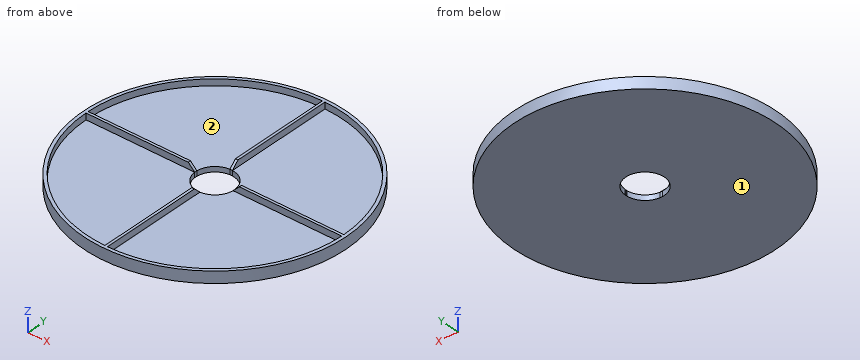
```python
from build123d import *

# Parameters (mm, degrees)
F1_DEPTH = 4
F0_R     = 102.5
F2_DEPTH = 9
F3_SIZE  = 5


with BuildPart() as f1:
    # F0 (on Top) → F1 (new body)
    with BuildSketch(Plane.XY):
        with BuildLine():
            Line((-1, -99.994999875), (-1, -14.9666295471))
            ThreePointArc((-1, -14.9666295471), (-10.6066017178, -10.6066017178), (-14.9666295471, -1))
            Line((-14.9666295471, -1), (-99.994999875, -1))
            ThreePointArc((-99.994999875, -1), (-70.7106781187, -70.7106781187), (-1, -99.994999875))
        make_face()
    extrude(amount=F1_DEPTH)



with BuildPart() as f1b:
    # F0 (on Top) → F1, piece 2 (new body)
    with BuildSketch(Plane.XY):
        with BuildLine():
            Line((99.994999875, -1), (14.9666295471, -1))
            ThreePointArc((14.9666295471, -1), (10.6066017178, -10.6066017178), (1, -14.9666295471))
            Line((1, -14.9666295471), (1, -99.994999875))
            ThreePointArc((1, -99.994999875), (70.7106781187, -70.7106781187), (99.994999875, -1))
        make_face()
    extrude(amount=F1_DEPTH)


with BuildPart() as f1c:
    # F0 (on Top) → F1, piece 3 (new body)
    with BuildSketch(Plane.XY):
        with BuildLine():
            ThreePointArc((1, 14.9666295471), (10.6066017178, 10.6066017178), (14.9666295471, 1))
            Line((14.9666295471, 1), (99.994999875, 1))
            ThreePointArc((99.994999875, 1), (70.7106781187, 70.7106781187), (1, 99.994999875))
            Line((1, 99.994999875), (1, 14.9666295471))
        make_face()
    extrude(amount=F1_DEPTH)


with BuildPart() as f1d:
    # F0 (on Top) → F1, piece 4 (new body)
    with BuildSketch(Plane.XY):
        with BuildLine():
            ThreePointArc((-14.9666295471, 1), (-10.6066017178, 10.6066017178), (-1, 14.9666295471))
            Line((-1, 14.9666295471), (-1, 99.994999875))
            ThreePointArc((-1, 99.994999875), (-70.7106781187, 70.7106781187), (-99.994999875, 1))
            Line((-99.994999875, 1), (-14.9666295471, 1))
        make_face()
    extrude(amount=F1_DEPTH)


with BuildPart() as f1_1:
    add(f1.part)

    add(f1b.part)  # F2 merges F1b

    add(f1c.part)  # F2 merges F1c

    add(f1d.part)  # F2 merges F1d
    # F0 (on Top) → F2 (join)
    with BuildSketch(Plane.XY):
        Circle(F0_R)
        with BuildLine():
            ThreePointArc((14.9666295471, 1), (14.9916550655, 0.5002783193), (15, 0))
            ThreePointArc((15, 0), (14.9916550655, -0.5002783193), (14.9666295471, -1))
            Line((14.9666295471, -1), (99.994999875, -1))
            ThreePointArc((99.994999875, -1), (70.7106781187, -70.7106781187), (1, -99.994999875))
            Line((1, -99.994999875), (1, -14.9666295471))
            ThreePointArc((1, -14.9666295471), (0, -15), (-1, -14.9666295471))
            Line((-1, -14.9666295471), (-1, -99.994999875))
            ThreePointArc((-1, -99.994999875), (-70.7106781187, -70.7106781187), (-99.994999875, -1))
            Line((-99.994999875, -1), (-14.9666295471, -1))
            ThreePointArc((-14.9666295471, -1), (-15, 0), (-14.9666295471, 1))
            Line((-14.9666295471, 1), (-99.994999875, 1))
            ThreePointArc((-99.994999875, 1), (-70.7106781187, 70.7106781187), (-1, 99.994999875))
            Line((-1, 99.994999875), (-1, 14.9666295471))
            ThreePointArc((-1, 14.9666295471), (0, 15), (1, 14.9666295471))
            Line((1, 14.9666295471), (1, 99.994999875))
            ThreePointArc((1, 99.994999875), (70.7106781187, 70.7106781187), (99.994999875, 1))
            Line((99.994999875, 1), (14.9666295471, 1))
        make_face(mode=Mode.SUBTRACT)
    extrude(amount=F2_DEPTH)

    # F3
    f3_edges = [f1_1.edges().sort_by_distance(p)[0] for p in [
        (0, -15, 9),
        (-15, 0, 9),
        (0, 15, 9),
        (15, 0, 9),
    ]]
    chamfer(f3_edges, length=F3_SIZE)


solid = f1_1.part
```
Verification items for the finished model (mm, model axes). Face numbers are marked on the shaded views. Round coordinates to 2 decimals unless told otherwise and drop trailing zeros. Write each loop counter-clockwise with the first axis right and the second up, starting at its lowest first coordinate (ties: lowest second). Pieces come first, ordered by that corner, then holes. Notation, with made-up numbers: (81, 43.5) - (102, 43.5) arc R18 cw to (102, 77.5) - close; hole circle Ø11 at (21.25, 55.5). An arc over 180 degrees is marked (long way). Answer as a JSON object with one key per item and string values. Group by question number.
Q1. Section check D-D, the plane x = 32. Enter the section's corners in (y, z), plus the area to 3 significant figures.
Q2. Mould release check, pull along X, two halves, no side actions. Record for the marked faces 1 and 2: released by +X, released by -X, zero draft, split by the parting line, or undercut.
Q3. Go/stop test with flat-tipped pins: pin 1 Ø2.5 at (x, z) = (54.5, 7) entering from -Y; pin 2 Ø4 at (y, z) = (47.5, 5) entering from +X; pin 3 Ø1.5 at (y, z) = (35.5, 7.5) entering from +X. Record where each tip stops, or that it passes through.
Q4. Section check B-B, the plane y = 89.5. Enter the section's corners in (x, z).
Q5. Section check A-A, the plane x = -12. Enter the section's corners in (y, z), plus the area to 3 significant figures.
Q6. Thickness scan on line 1 (X direction, y = 79.5, z = 7.5); line 2 (Y direction, x = -31, z = 6); line 3 (Y direction, x = 65, z = 4.5). Record the ranges inside material, lowest first.
Q7. Section check C-C, the plane z = 5.75. Enter the section's corners in (x, y) (3 decimals), plus the area to 3 significant figures.
Found:
{
 "1": {"outline": "(-97.38, 0) - (97.38, 0) - (97.38, 9) - (94.74, 9) - (94.74, 4) - (1, 4) - (1, 9) - (-1, 9) - (-1, 4) - (-94.74, 4) - (-94.74, 9) - (-97.38, 9) - close", "area": "815 mm^2"},
 "2": {"face 1": "zero draft", "face 2": "undercut"},
 "3": {"pin 1": "stops at y = -87.58", "pin 2": "stops at x = 91.85", "pin 3": "stops at x = 96.43"},
 "4": {"outline": "(-49.96, 0) - (49.96, 0) - (49.96, 9) - (44.61, 9) - (44.61, 4) - (1, 4) - (1, 9) - (-1, 9) - (-1, 4) - (-44.61, 4) - (-44.61, 9) - (-49.96, 9) - close"},
 "5": {"outline": "(-101.8, 0) - (-9, 0) - (-9, 4) - (-99.28, 4) - (-99.28, 9) - (-101.8, 9) - close; (9, 0) - (101.8, 0) - (101.8, 9) - (99.28, 9) - (99.28, 4) - (9, 4) - close", "area": "768 mm^2"},
 "6": {"line 1": "x = -64.7 to -60.66, -1 to 1, 60.66 to 64.7", "line 2": "y = -97.7 to -95.07, -1 to 1, 95.07 to 97.7", "line 3": "y = -79.25 to -75.99, -1 to 1, 75.99 to 79.25"},
 "7": {"outline": "circle Ø205 at (0, 0); hole (-99.995, -1) arc R100 ccw to (-1, -99.995) - (-1, -16.72) arc R16.75 ccw to (1, -16.72) - (1, -99.995) arc R100 ccw to (99.995, -1) - (16.72, -1) arc R16.75 ccw to (16.72, 1) - (99.995, 1) arc R100 ccw to (1, 99.995) - (1, 16.72) arc R16.75 ccw to (-1, 16.72) - (-1, 99.995) arc R100 ccw to (-99.995, 1) - (-16.72, 1) arc R16.75 ccw to (-16.72, -1) - close", "area": "2,260 mm^2"}
}
